Verification items for this drawing (mm, ordinates from the low corner). A direction names the side the tool comes from. Give positions to 0.01 mm unless a question says otherwise; leave off trailing zeros. Write each loop counter-clockwise with the first axis right and the second up, starting at its lowest first coordinate (ties: lowest second). Pieces come first, ordered by that corner, then holes. Notation, with made-up numbers: (-11, -29.5) -> (27, -29.5) arc R27 cw to (27, 3.5) -> close; hole circle Ø1 at (59.5, 4). An arc over 180 degrees is marked (long way). One line per item, written item: value.
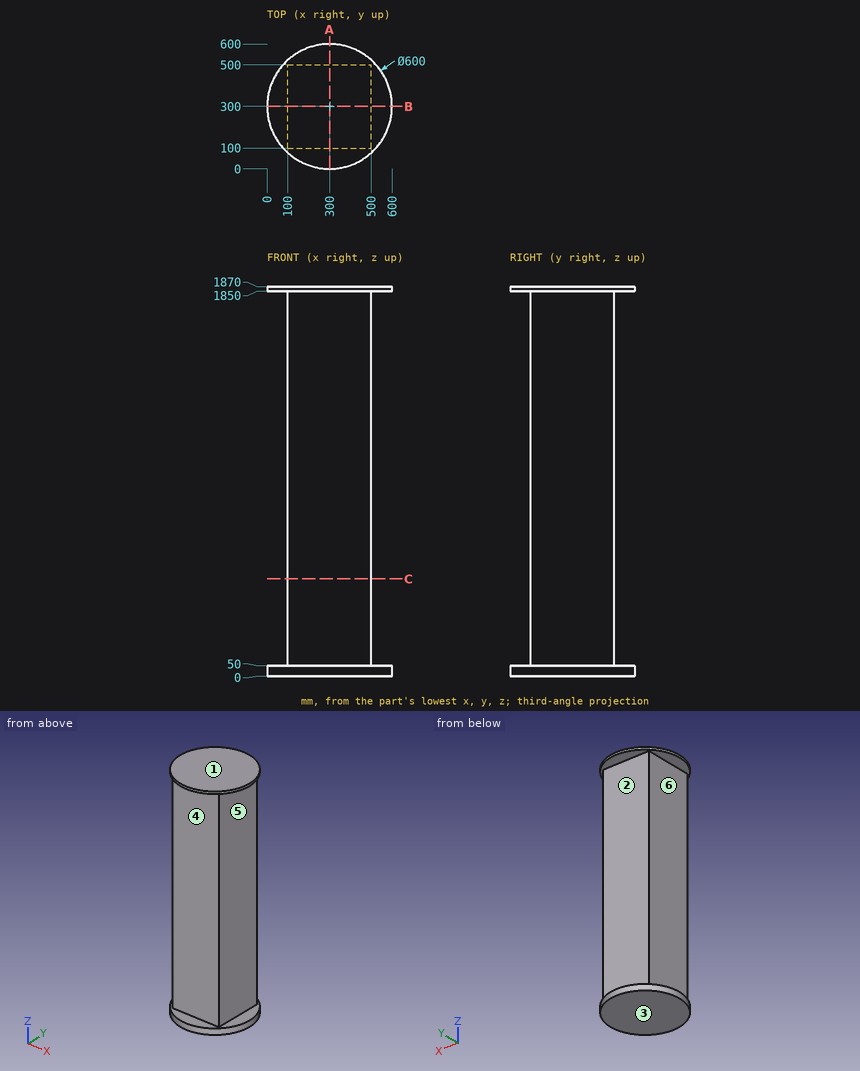
1) Sectioned sample at C-C on z = 467. Record the cut outline in (x, y).
Verdict:
outline: (100, 100) -> (500, 100) -> (500, 500) -> (100, 500) -> close
2) Sectioned sample at A-A on x = 300. Record the cut outline in (y, z), plus the area to 3 significant figures.
Verdict:
outline: (0, 0) -> (600, 0) -> (600, 50) -> (500, 50) -> (500, 1850) -> (600, 1850) -> (600, 1870) -> (0, 1870) -> (0, 1850) -> (100, 1850) -> (100, 50) -> (0, 50) -> close
area: 762,000 mm^2
3) Tool access check on the marked faces 4, 5 and 6. Record the directions out of +Z, -Z, +X, -X, +Y, -Y that give a thin tool (end or side, any length) a straight path to the whole face; none if there is none.
Verdict:
face 4: +X, -X, -Y
face 5: +X, +Y, -Y
face 6: -X, +Y, -Y
4) Mould release check, pull along Z, two halves, no side actions. Record for the marked faces 1, 2 and 3: released by +Z, released by -Z, zero draft, split by the parting line, or undercut.
Verdict:
face 1: released by +Z
face 2: undercut
face 3: released by -Z
5) Scan lines: probe 1 along Z at (x, y) = (511.5, 312); probe 2 along Y at (x, z) = (377, 156). Record each from-to range of solid material in increasing order.
Verdict:
probe 1: 0 to 50, 1850 to 1870
probe 2: 100 to 500
6) Depth check by flat-ended pin: pin 1 Ø12 at (x, z) = (233, 1603) entering from -Y; pin 2 Ø12 at (y, z) = (464.5, 1492.5) entering from +X; pin 3 Ø6 at (x, z) = (117, 731) entering from +Y. Enter the tip coordinate at first touch or a pass-through.
Verdict:
pin 1: y = 100
pin 2: x = 500
pin 3: y = 500
